```python
from build123d import *

# Parameters (mm, degrees)
BOSS_EXTRUDE1_DEPTH         = 4.7625
CUT_EXTRUDE1_DEPTH          = 198.884278841
FILLET1_R                   = 3.175
FILLET2_R                   = 9.525
F_12_0_189_DIAMETER_HOLE1_D = 4.8006
F_8_CLEARANCE_HOLE1_D       = 4.4958
FILLET3_RADIUS              = 2.38125
FILLET3_LENGTH              = 15.875
FILLET4_RADIUS              = 2.38125
FILLET4_LENGTH              = 15.875
FILLET5_RADIUS              = 2.38125
FILLET5_LENGTH              = 15.875
FILLET6_START               = -17
FILLET6_DEPTH               = 19


with BuildPart() as part:
    # Sketch1 → Boss-Extrude1 (new body)
    with BuildSketch(Plane.XY):
        Polygon((0, 0), (9.525, 0), (9.525, -15.875), (30.1625, -15.875), (30.1625, 0), (39.6875, 0), (39.6875, -15.875), (182.5625, -15.875), (182.5625, 0), (-16.893133293, 76.2), align=None)
    extrude(amount=BOSS_EXTRUDE1_DEPTH)

    # Sketch2 → Cut-Extrude1 (cut, through all)
    with BuildSketch(Plane.XY.offset(4.7625)):
        Polygon((7.644620712, 9.525), (130.941072945, 9.525), (-3.76442223, 60.987867019), align=None)
    extrude(amount=-CUT_EXTRUDE1_DEPTH, mode=Mode.SUBTRACT)

    # Fillet1
    fillet1_edges = [part.edges().sort_by_distance(p)[0] for p in [
        (7.644620712, 9.525, 2.38125),
        (-3.76442223, 60.987867019, 2.38125),
        (130.941072945, 9.525, 2.38125),
    ]]
    fillet(fillet1_edges, radius=FILLET1_R)

    # Fillet2
    fillet2_edges = [part.edges().sort_by_distance(p)[0] for p in [
        (-16.893133293, 76.2, 2.38125),
    ]]
    fillet(fillet2_edges, radius=FILLET2_R)

    # #12 (0.189) Diameter Hole1 (through all)
    with Locations(Plane.XY.offset(4.7625)):
        with Locations((-5.72515333, 63.259750533), (2.244424524, 11.879883041)):
            Hole(F_12_0_189_DIAMETER_HOLE1_D / 2)

    # #8 Clearance Hole1 (through all)
    with Locations(Plane.XY.offset(4.7625)):
        with Locations((19.84375, -11.1125), (52.3875, -11.1125), (169.8625, -11.1125)):
            Hole(F_8_CLEARANCE_HOLE1_D / 2)

    # Fillet3: full round fillet: the end face becomes a half cylinder, R = half its width
    fillet3_face = Plane((9.525, -7.9375, 2.38125), x_dir=(0, 1, 0), z_dir=(-1, 0, 0))  # on the end face: x along it, z out of the body
    fillet3_slab = fillet3_face.offset(-FILLET3_RADIUS / 2) * Box(FILLET3_LENGTH, 2 * FILLET3_RADIUS, FILLET3_RADIUS, mode=Mode.PRIVATE)  # the body's end, R deep
    fillet3_round = Plane((11.90625, -7.9375, 2.38125), x_dir=(-1, 0, 0), z_dir=(0, 1, 0)) * Cylinder(FILLET3_RADIUS, FILLET3_LENGTH, mode=Mode.PRIVATE)  # its axis R under the face
    add(fillet3_slab - fillet3_round, mode=Mode.SUBTRACT)

    # Fillet4: full round fillet: the end face becomes a half cylinder, R = half its width
    fillet4_face = Plane((30.1625, -7.9375, 2.38125), x_dir=(0, 1, 0), z_dir=(1, 0, 0))  # on the end face: x along it, z out of the body
    fillet4_slab = fillet4_face.offset(-FILLET4_RADIUS / 2) * Box(FILLET4_LENGTH, 2 * FILLET4_RADIUS, FILLET4_RADIUS, mode=Mode.PRIVATE)  # the body's end, R deep
    fillet4_round = Plane((27.78125, -7.9375, 2.38125), x_dir=(1, 0, 0), z_dir=(0, 1, 0)) * Cylinder(FILLET4_RADIUS, FILLET4_LENGTH, mode=Mode.PRIVATE)  # its axis R under the face
    add(fillet4_slab - fillet4_round, mode=Mode.SUBTRACT)

    # Fillet5: full round fillet: the end face becomes a half cylinder, R = half its width
    fillet5_face = Plane((39.6875, -7.9375, 2.38125), x_dir=(0, -1, 0), z_dir=(-1, 0, 0))  # on the end face: x along it, z out of the body
    fillet5_slab = fillet5_face.offset(-FILLET5_RADIUS / 2) * Box(FILLET5_LENGTH, 2 * FILLET5_RADIUS, FILLET5_RADIUS, mode=Mode.PRIVATE)  # the body's end, R deep
    fillet5_round = Plane((42.06875, -7.9375, 2.38125), x_dir=(-1, 0, 0), z_dir=(0, -1, 0)) * Cylinder(FILLET5_RADIUS, FILLET5_LENGTH, mode=Mode.PRIVATE)  # its axis R under the face
    add(fillet5_slab - fillet5_round, mode=Mode.SUBTRACT)

    # Fillet6: read off the stored shape, not the designer's step
    # Fillet6 outline → Fillet6 (cut)
    with BuildSketch(Plane(origin=(0, 0, 0), x_dir=(1, 0, 0), z_dir=(0, 1, 0)).offset(FILLET6_START)):
        with BuildLine():
            ThreePointArc((180.18125, 0), (181.865048023, -0.697451977), (182.5625, -2.38125))
            Line((182.5625, -2.38125), (182.5625, 0))
            Line((182.5625, 0), (180.18125, 0))
        make_face()
        with BuildLine():
            ThreePointArc((182.5625, -2.38125), (181.865048023, -4.065048023), (180.18125, -4.7625))
            Line((180.18125, -4.7625), (182.5625, -4.7625))
            Line((182.5625, -4.7625), (182.5625, -2.38125))
        make_face()
    extrude(amount=FILLET6_DEPTH, mode=Mode.SUBTRACT)


solid = part.part
```
Could you check a few things on this model? Use its own coordinates, in mm. A direction names the side the tool comes from. Round coordinates to 2 decimals unless told otherwise and drop trailing zeros. Loops run counter-clockwise (first coordinate to the right, second up) from the corner with the lowest first, then second, coordinate; pieces in that order, holes last. Notation, with made-up numbers: (80.25, 78) -> (132.25, 78) arc R17 ccw to (132.25, 90) -> close; hole circle Ø9 at (89.25, -9.75). An arc over 180 degrees is marked (long way). Put each result on its own line as item: value.
Q1. I want a section at C-C on y = 36. Write out the boundary of the cut face in (x, z), and give its area (3 significant figures).
Checks:
outline: (-7.98, 0) -> (1.78, 0) -> (1.78, 4.76) -> (-7.98, 4.76) -> close; (61.64, 0) -> (88.33, 0) -> (88.33, 4.76) -> (61.64, 4.76) -> close
area: 174 mm2
Q2. Thinking about a two-plate mould opening in X: for faces 6 (the flat face through (2.236, 33.924, 2.415)), 7 (the flat face through (92.379, 34.454, 2.348)), 8 (the flat face through (110, -15.875, 2)), which applies, pulls with the +X half, pulls with the -X half, needs draft (parallel to the pull), parting line crosses it, or undercut?
Checks:
face 6: undercut
face 7: pulls with the +X half
face 8: needs draft
Q3. I want a section at A-A on x = 20. Write out the boundary of the cut face in (y, z) (1 decimal).
Checks:
outline: (-15.9, 0) -> (-13.4, 0) -> (-13.4, 4.8) -> (-15.9, 4.8) -> close; (-8.9, 0) -> (9.5, 0) -> (9.5, 4.8) -> (-8.9, 4.8) -> close; (51.9, 0) -> (62.1, 0) -> (62.1, 4.8) -> (51.9, 4.8) -> close
Q4. Please list where these lines run through material, in increasing order: line 1 (X direction, y = -8, z = 2.05); line 2 (Y direction, x = 42.5, z = 1.75) (3 decimals); line 3 (Y direction, x = 171, z = 2.1) (3 decimals). Write a range as from..to.
Checks:
line 1: 9.55..30.14, 39.71..182.54
line 2: -15.875..9.525, 43.313..53.509
line 3: -15.875..-13.051, -9.174..4.417
Q5. I want a section at B-B on z = 3.1. Give the number of separate pieces and of enclosed holes in the cut face, and give its area (3 significant figures).
Checks:
separate pieces: 1
enclosed holes: 6
area: 6,270 mm2
Q6. For pin 1 Ø3 at (x, y) = (2.24, 11.88) entering from +Z (3 decimals); pin 2 Ø2 at (y, z) = (14.5, 1) entering from -X; pin 3 Ø1.5 at (x, z) = (154.5, 3) entering from +Y, each with a flat end and sliding along its axis, tell me the tip position at first contact or that it passes through.
Checks:
pin 1: through
pin 2: x = -3.44
pin 3: y = 11.01
Q7. I want a section at D-D on x = 45. Write out the boundary of the cut face in (y, z) (1 decimal).
Checks:
outline: (-15.9, 0) -> (9.5, 0) -> (9.5, 4.8) -> (-15.9, 4.8) -> close; (42.4, 0) -> (52.6, 0) -> (52.6, 4.8) -> (42.4, 4.8) -> close
Q8. Which directions (+Z, -Z, +X, -X, +Y, -Y) give clear straight access to the entire face, cutting with the end or side of a thin tool? Please do faces 1 (the flat face through (20, -15.875, 2)), 2 (the cylindrical face through (39.688, -8.049, 2.434)), 3 (the cylindrical face through (9.526, -7.826, 2.329)), 4 (the flat face through (-6.623, 29.876, 2.348)), 5 (the flat face through (59.1, 36.97, 2.41)).
Checks:
face 1: +Z, -Z, +X, -X, -Y
face 2: -Y
face 3: -X, -Y
face 4: +Z, -Z, -X, -Y
face 5: +Z, -Z
